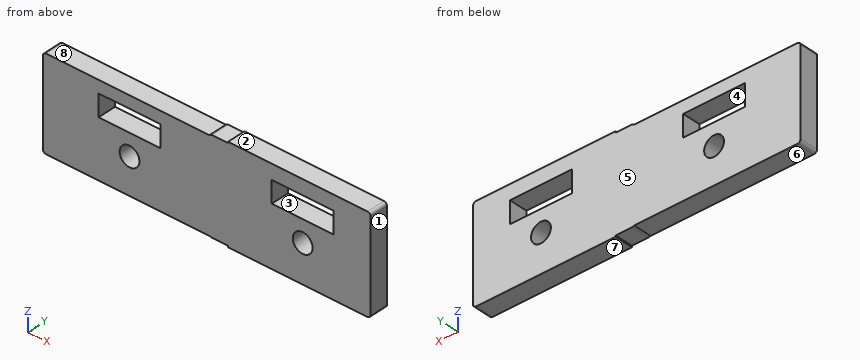
```python
from build123d import *

# Parameters (mm, degrees)
CROQUIS1_W              = 150
CROQUIS1_H              = 30
SALIENTE_EXTRUIR1_DEPTH = 3
CROQUIS2_R              = 1.6
CROQUIS2_W              = 10
CROQUIS2_H              = 3.5
CORTAR_EXTRUIR1_DEPTH   = 77.544104933
CORTAR_EXTRUIR2_START   = -10
CROQUIS3_R              = 1.6
CROQUIS3_W              = 10
CROQUIS3_H              = 3.5
CORTAR_EXTRUIR2_DEPTH   = 10
CROQUIS4_W              = 26.059818974
CROQUIS4_H              = 3
SALIENTE_EXTRUIR2_DEPTH = 0.2
CROQUIS6_W              = 23.059818974
CROQUIS6_H              = 3
SALIENTE_EXTRUIR4_DEPTH = 0.2
CROQUIS7_W              = 23.059818974
CROQUIS7_H              = 3
SALIENTE_EXTRUIR5_DEPTH = 0.2
REDONDEO1_R             = 0.5


with BuildPart() as part:
    # Croquis1 → Saliente-Extruir1 (new body)
    with BuildSketch(Plane(origin=(0, 0, 0), x_dir=(1, 0, 0), z_dir=(0, 1, 0))):
        Rectangle(CROQUIS1_W, CROQUIS1_H)
    extrude(amount=SALIENTE_EXTRUIR1_DEPTH)

    # Croquis2 → Cortar-Extruir1 (cut, through all)
    with BuildSketch(Plane(origin=(0, 3, 0), x_dir=(1, 0, 0), z_dir=(0, 1, 0))):
        with Locations(Location((61, -6, 0), (0, 0, 270))):
            Circle(CROQUIS2_R)
        with Locations(Location((33, -6, 0), (0, 0, 270))):
            Circle(CROQUIS2_R)
        with Locations(Location((-33, -6, 0), (0, 0, 90))):
            Circle(CROQUIS2_R)
        with Locations(Location((-61, -6, 0), (0, 0, 90))):
            Circle(CROQUIS2_R)
        with Locations((61, -11.25)):
            Rectangle(CROQUIS2_W, CROQUIS2_H)
        with Locations((33, -11.25)):
            Rectangle(CROQUIS2_W, CROQUIS2_H)
        with Locations((-33, -11.25)):
            Rectangle(CROQUIS2_W, CROQUIS2_H)
        with Locations((-61, -11.25)):
            Rectangle(CROQUIS2_W, CROQUIS2_H)
    extrude(amount=-CORTAR_EXTRUIR1_DEPTH, mode=Mode.SUBTRACT)

    # Croquis3 → Cortar-Extruir2 (cut)
    with BuildSketch(Plane.XZ.offset(CORTAR_EXTRUIR2_START)):
        Polygon((-48.06783131, 0.2), (-75, 0.2), (-75, -15), (75, -15), (75, 15), (-22.008012336, 15), (-22.008012336, 0.1), (-48.06783131, 0.1), align=None)
        with Locations((33, 6)):
            Circle(CROQUIS3_R, mode=Mode.SUBTRACT)
        with Locations((61, 6)):
            Circle(CROQUIS3_R, mode=Mode.SUBTRACT)
        with Locations((33, 11.25)):
            Rectangle(CROQUIS3_W, CROQUIS3_H, mode=Mode.SUBTRACT)
        with Locations((61, 11.25)):
            Rectangle(CROQUIS3_W, CROQUIS3_H, mode=Mode.SUBTRACT)
    extrude(amount=CORTAR_EXTRUIR2_DEPTH, mode=Mode.SUBTRACT)

    # Croquis4 → Saliente-Extruir2 (add)
    with BuildSketch(Plane.XY.offset(15)):
        with Locations((-35.037921823, 1.5)):
            Rectangle(CROQUIS4_W, CROQUIS4_H)
    extrude(amount=SALIENTE_EXTRUIR2_DEPTH)

    # Croquis6 → Saliente-Extruir4 (add)
    with BuildSketch(Plane(origin=(0, 0, 0.1), x_dir=(-1, 0, 0), z_dir=(0, 0, -1))):
        with Locations((33.537921823, 1.5)):
            Rectangle(CROQUIS6_W, CROQUIS6_H)
    extrude(amount=SALIENTE_EXTRUIR4_DEPTH)

    # Croquis7 → Saliente-Extruir5 (add)
    with BuildSketch(Plane.XY.offset(15.2)):
        with Locations((-33.537921823, 1.5)):
            Rectangle(CROQUIS7_W, CROQUIS7_H)
    extrude(amount=SALIENTE_EXTRUIR5_DEPTH)

    # Redondeo1
    # the kernel refuses this fillet: 0.5 mm, written as the material it takes off along each edge
    with BuildSketch(Plane(origin=(-48.06783131, 3.75, 0.1), x_dir=(0, 0, 1), z_dir=(0, -1, 0))) as redondeo1_piece_1:
        with BuildLine():
            CenterArc((0.5, -0.3), REDONDEO1_R, 143.130102354, 36.869897646)
            Line((0, -0.3), (-0.01, -0.3))
            Line((-0.01, -0.3), (-0.01, 0))
            Line((-0.01, 0), (0, 0.01))
            ThreePointArc((0, 0.01), (0.05, 0.01), (0.092, 0.006))
            Line((0.092, 0.006), (0.1, 0))
        make_face()
    extrude(amount=4.5, mode=Mode.SUBTRACT)
    with BuildSketch(Plane(origin=(-48.06783131, -1, 15.2), x_dir=(1, 0, 0), z_dir=(0, 1, 0))) as redondeo1_piece_2:
        with BuildLine():
            CenterArc((0.4, 0.5), REDONDEO1_R, 216.869897645, 53.130102355)
            Line((0, 0.2), (-0.008, 0.194))
            ThreePointArc((-0.008, 0.194), (-0.01, 0.1), (-0.01, 0))
            Line((-0.01, 0), (0, -0.01))
            Line((0, -0.01), (0.4, -0.01))
            Line((0.4, -0.01), (0.4, 0))
        make_face()
    extrude(amount=5, mode=Mode.SUBTRACT)
    with BuildSketch(Plane(origin=(-22.008012336, -1.25, 15.4), x_dir=(0, 0, -1), z_dir=(0, 1, 0)), Plane(origin=(-75, -1.25, 15), x_dir=(1, 0, 0), z_dir=(0, 1, 0))) as redondeo1_piece_3:
        with BuildLine():
            CenterArc((REDONDEO1_R, REDONDEO1_R), REDONDEO1_R, 180, 90)
            Line((0, REDONDEO1_R), (-REDONDEO1_R * 0.02, REDONDEO1_R))
            Line((-REDONDEO1_R * 0.02, REDONDEO1_R), (-REDONDEO1_R * 0.02, -REDONDEO1_R * 0.02))
            Line((-REDONDEO1_R * 0.02, -REDONDEO1_R * 0.02), (REDONDEO1_R, -REDONDEO1_R * 0.02))
            Line((REDONDEO1_R, -REDONDEO1_R * 0.02), (REDONDEO1_R, 0))
        make_face()
    extrude(amount=5.5, mode=Mode.SUBTRACT)
    with BuildSketch(Plane(origin=(-22.008012336, 4.25, -0.1), x_dir=(-1, 0, 0), z_dir=(0, -1, 0)), Plane(origin=(-75, 4.25, 0.2), x_dir=(0, 0, 1), z_dir=(0, -1, 0))) as redondeo1_piece_4:
        with BuildLine():
            CenterArc((REDONDEO1_R, -REDONDEO1_R), REDONDEO1_R, 90, 90)
            Line((0, -REDONDEO1_R), (-REDONDEO1_R * 0.02, -REDONDEO1_R))
            Line((-REDONDEO1_R * 0.02, -REDONDEO1_R), (-REDONDEO1_R * 0.02, REDONDEO1_R * 0.02))
            Line((-REDONDEO1_R * 0.02, REDONDEO1_R * 0.02), (REDONDEO1_R, REDONDEO1_R * 0.02))
            Line((REDONDEO1_R, REDONDEO1_R * 0.02), (REDONDEO1_R, 0))
        make_face()
    extrude(amount=5.5, mode=Mode.SUBTRACT)


solid = part.part
```
Work out the finished part from the listing and answer in its coordinate system (mm). Face numbers are marked on the shaded views. A direction names the side the tool comes from. Give positions to 0.01 mm unless a question says otherwise; leave off trailing zeros. Write each loop counter-clockwise with the first axis right and the second up, starting at its lowest first coordinate (ties: lowest second). Pieces come first, ordered by that corner, then holes. Notation, with made-up numbers: (80.25, 77) -> (98.25, 77) arc R30 ccw to (98.25, 116) -> close; hole circle Ø2 at (-33.5, -5.75). An arc over 180 degrees is marked (long way). Write item = value, one per line.
Q1. Section D-D on x = -53.5 is taken. Determine the outline of the cut face in (y, z), and give its area (3 significant figures).
Computed values:
outline = (0, 0.2) -> (3, 0.2) -> (3, 15) -> (0, 15) -> close
area = 44.4 mm^2
Q2. Section B-B on z = 6 is taken. Determine the outline of the cut face in (x, y), and give its area (3 significant figures).
Computed values:
outline = (-75, 0) -> (-62.6, 0) -> (-62.6, 3) -> (-75, 3) -> close; (-59.4, 0) -> (-34.6, 0) -> (-34.6, 3) -> (-59.4, 3) -> close; (-31.4, 0) -> (-22.01, 0) -> (-22.01, 3) -> (-31.4, 3) -> close
area = 140 mm^2
Q3. Section C-C on y = 2 is taken. Determine the outline of the cut face in (x, z).
Computed values:
outline = (-75, 0.7) arc R0.5 ccw to (-74.5, 0.2) -> (-48.07, 0.2) arc R0.5 ccw to (-47.77, 0.1) -> (-45.07, 0.1) -> (-45.07, -0.1) -> (-22.51, -0.1) arc R0.5 ccw to (-22.01, 0.4) -> (-22.01, 14.9) arc R0.5 ccw to (-22.51, 15.4) -> (-45.07, 15.4) -> (-45.07, 15.2) -> (-47.67, 15.2) arc R0.5 ccw to (-48.07, 15) -> (-74.5, 15) arc R0.5 ccw to (-75, 14.5) -> close; hole (-66, 9.5) -> (-56, 9.5) -> (-56, 13) -> (-66, 13) -> close; hole circle Ø3.2 at (-61, 6); hole (-38, 9.5) -> (-28, 9.5) -> (-28, 13) -> (-38, 13) -> close; hole circle Ø3.2 at (-33, 6)
Q4. Flat-ended cylindrical pins translate along their axes: pin 1 Ø0.9 at (x, y) = (-61.5, 2) entering from -Z; pin 2 Ø8 at (x, z) = (-52, 12) entering from -Y; pin 3 Ø1.4 at (x, y) = (-46.5, 1) entering from -Z. Find the tip coordinate at first contact, or state that the pin passes through.
Computed values:
pin_1 = 0.2
pin_2 = 0
pin_3 = 0.1
Q5. Section A-A on x = -33 is taken. Determine the outline of the cut face in (y, z), and give its area (3 significant figures).
Computed values:
outline = (0, -0.1) -> (3, -0.1) -> (3, 4.4) -> (0, 4.4) -> close; (0, 7.6) -> (3, 7.6) -> (3, 9.5) -> (0, 9.5) -> close; (0, 13) -> (3, 13) -> (3, 15.4) -> (0, 15.4) -> close
area = 26.4 mm^2
Q6. A tool of negligible diameter and unlimited length cuts with its end or side. For the marked faces 4, 5, 6, 7 and 8, from which of +Z, -Z, +X, -X, +Y, -Y can it reach the whole face along a straight path? Write none if from no direction.
Computed values:
face_4 = +Y, -Y
face_5 = +Z, -Z, +X, -X, +Y
face_6 = -Z, -X, +Y, -Y
face_7 = -Z, +X, -X, +Y, -Y
face_8 = +Z, -X, +Y, -Y
Q7. Consider line 1 along X through (y, z) = (1.6, 6); line 2 along Z through (x, y) = (-33, 1.4); line 3 along Z through (x, y) = (-61, 1.7). Determine where each line is inside the solid, lowest interval first.
Computed values:
line_1 = -75 to -62.6, -59.4 to -34.6, -31.4 to -22.01
line_2 = -0.1 to 4.4, 7.6 to 9.5, 13 to 15.4
line_3 = 0.2 to 4.4, 7.6 to 9.5, 13 to 15
Q8. For a pull along X with two mould halves and no side action, classify the marked faces 1, 2 and 3 as pulls with the +X half, pulls with the -X half, needs draft (parallel to the pull), parting line crosses it, or undercut.
Computed values:
face_1 = pulls with the +X half
face_2 = needs draft
face_3 = undercut
